Can you work these out from the model? Positions are in its coordinate system, mm. Face numbers are marked on the shaded views. A direction names the side the tool comes from. Round coordinates to 2 decimals unless told otherwise and drop trailing zeros. Write each loop counter-clockwise with the first axis right and the second up, starting at its lowest first coordinate (ties: lowest second). Pieces come first, ordered by that corner, then holes. Notation, with made-up numbers: M 88.25,-16 L 123.25,-16 A26 cw 123.25,8 Z; hole C 45.25,61 d4. An arc over 180 degrees is marked long. Answer in a Markdown table with one row per item. Add a question column.
(1) Suppose I cut it at B-B, the plane x = 3.5. Write out the boundary of the cut face in (y, z).
(2) If we mould it in two halves opening along Y, with no side actions, what happens to the marked faces 3, 4 and 5? For each: released by +Y, released by -Y, zero draft, split by the parting line, or undercut.
(3) I'm going to push flat-ended pins straight in: pin 1 (5.5 mm diameter, centred on x = 5, z = 28.5, fed in from +Y); pin 2 (10 mm diameter, centred on x = 29.5, z = 59.5, fed in from +Y); pin 3 (4 mm diameter, centred on y = 51, z = 30.5, fed in from +X); pin 4 (14 mm diameter, centred on x = 5.5, y = 52, fed in from -Z). Where does each tip first touch, or does it pass through?
(4) Suppose I cut it at C-C, the plane y = 37.5. Write out the boundary of the cut face in (x, z), then the cut area to 3 significant figures.
(5) For the marked faces 1 and 2, which set-ups out of +Z, -Z, +X, -X, +Y, -Y let a thin tool reach every point of the face, with its end or its side?
(6) If I drill on probe 1 along Z at (x, y) = (9.5, 28); probe 2 along X at (y, z) = (7, 19); probe 3 along Z at (x, y) = (7.5, 51), over which ranges is the centre line in solid material (lowest first)?
(7) Suppose I cut it at D-D, the plane x = 34. Write out the boundary of the cut face in (y, z).
(8) Suppose I cut it at A-A, the plane z = 31.5. Write out the boundary of the cut face in (x, y), then the cut area to 3 significant figures.
from build123d import *

# Parameters (mm, degrees)
SKETCH1_W           = 57.15
SKETCH1_H           = 57.15
BOSS_EXTRUDE1_DEPTH = 55.118
SKETCH2_R           = 19.05
BOSS_EXTRUDE2_DEPTH = 1.524
SKETCH3_R           = 3.175
BOSS_EXTRUDE3_DEPTH = 19.05
SKETCH18_W          = 20.32
SKETCH18_H          = 20.32
CUT_EXTRUDE13_DEPTH = 50.038
SKETCH20_W          = 20.32
SKETCH20_H          = 20.32
CUT_EXTRUDE14_DEPTH = 50.038
SKETCH21_W          = 20.32
SKETCH21_H          = 20.32
CUT_EXTRUDE15_DEPTH = 50.038
SKETCH22_W          = 20.32
SKETCH22_H          = 20.32
CUT_EXTRUDE16_DEPTH = 50.038
SKETCH11_R          = 2.54
CUT_EXTRUDE8_DEPTH  = 98.827597967
SKETCH12_R          = 2.54
CUT_EXTRUDE9_DEPTH  = 98.827597967
SKETCH14_R          = 2.54
CUT_EXTRUDE10_DEPTH = 98.827597967
SKETCH15_R          = 2.54
CUT_EXTRUDE11_DEPTH = 98.827597967
FILLET2_R           = 5.08
FILLET4_R           = 2.54
FILLET1_R           = 0.508
SKETCH10_W          = 7.148953117
SKETCH10_H          = 1.106198654
CUT_EXTRUDE7_DEPTH  = 14.986


with BuildPart() as part:
    # Sketch1 → Boss-Extrude1 (new body)
    with BuildSketch(Plane.XY):
        with Locations((28.575, 28.575)):
            Rectangle(SKETCH1_W, SKETCH1_H)
    extrude(amount=BOSS_EXTRUDE1_DEPTH)

    # Sketch2 → Boss-Extrude2 (add)
    with BuildSketch(Plane.XY.offset(55.118)):
        with Locations(Location((28.575, 28.575, 0), (0, 0, 180))):
            Circle(SKETCH2_R)
    extrude(amount=BOSS_EXTRUDE2_DEPTH)

    # Sketch3 → Boss-Extrude3 (add)
    with BuildSketch(Plane.XY.offset(56.642)):
        with Locations(Location((28.575, 28.575, 0), (0, 0, 180))):
            Circle(SKETCH3_R)
    extrude(amount=BOSS_EXTRUDE3_DEPTH)

    # Sketch18 → Cut-Extrude13 (cut)
    with BuildSketch(Plane(origin=(0, 0, 0), x_dir=(-1, 0, 0), z_dir=(0, 0, -1))):
        with Locations((0, 57.15)):
            Rectangle(SKETCH18_W, SKETCH18_H)
    extrude(amount=-CUT_EXTRUDE13_DEPTH, mode=Mode.SUBTRACT)

    # Sketch20 → Cut-Extrude14 (cut)
    with BuildSketch(Plane(origin=(0, 0, 0), x_dir=(-1, 0, 0), z_dir=(0, 0, -1))):
        Rectangle(SKETCH20_W, SKETCH20_H)
    extrude(amount=-CUT_EXTRUDE14_DEPTH, mode=Mode.SUBTRACT)

    # Sketch21 → Cut-Extrude15 (cut)
    with BuildSketch(Plane(origin=(0, 0, 0), x_dir=(-1, 0, 0), z_dir=(0, 0, -1))):
        with Locations((-57.15, 0)):
            Rectangle(SKETCH21_W, SKETCH21_H)
    extrude(amount=-CUT_EXTRUDE15_DEPTH, mode=Mode.SUBTRACT)

    # Sketch22 → Cut-Extrude16 (cut)
    with BuildSketch(Plane(origin=(0, 0, 0), x_dir=(-1, 0, 0), z_dir=(0, 0, -1))):
        with Locations((-57.15, 57.15)):
            Rectangle(SKETCH22_W, SKETCH22_H)
    extrude(amount=-CUT_EXTRUDE16_DEPTH, mode=Mode.SUBTRACT)

    # Sketch11 → Cut-Extrude8 (cut, through all)
    with BuildSketch(Plane.XY.offset(55.118)):
        with Locations((4.953, 52.233071325)):
            Circle(SKETCH11_R)
    extrude(amount=-CUT_EXTRUDE8_DEPTH, mode=Mode.SUBTRACT)

    # Sketch12 → Cut-Extrude9 (cut, through all)
    with BuildSketch(Plane.XY.offset(55.118)):
        with Locations((52.197, 52.233071325)):
            Circle(SKETCH12_R)
    extrude(amount=-CUT_EXTRUDE9_DEPTH, mode=Mode.SUBTRACT)

    # Sketch14 → Cut-Extrude10 (cut, through all)
    with BuildSketch(Plane.XY.offset(55.118)):
        with Locations((4.953, 4.989071325)):
            Circle(SKETCH14_R)
    extrude(amount=-CUT_EXTRUDE10_DEPTH, mode=Mode.SUBTRACT)

    # Sketch15 → Cut-Extrude11 (cut, through all)
    with BuildSketch(Plane.XY.offset(55.118)):
        with Locations((52.197, 4.989071325)):
            Circle(SKETCH15_R)
    extrude(amount=-CUT_EXTRUDE11_DEPTH, mode=Mode.SUBTRACT)

    # Fillet2
    fillet2_edges = [part.edges().sort_by_distance(p)[0] for p in [
        (0, 57.15, 52.578),
        (57.15, 57.15, 52.578),
        (57.15, 0, 52.578),
        (0, 0, 52.578),
    ]]
    fillet(fillet2_edges, radius=FILLET2_R)

    # Fillet4
    fillet4_edges = [part.edges().sort_by_distance(p)[0] for p in [
        (0, 28.575, 0),
        (10.16, 52.07, 0),
        (5.08, 46.99, 0),
        (0, 46.99, 25.019),
        (10.16, 57.15, 25.019),
        (10.16, 46.99, 25.019),
        (28.575, 0, 0),
        (5.08, 10.16, 0),
        (10.16, 5.08, 0),
        (10.16, 0, 25.019),
        (0, 10.16, 25.019),
        (10.16, 10.16, 25.019),
        (57.15, 28.575, 0),
        (46.99, 5.08, 0),
        (52.07, 10.16, 0),
        (57.15, 10.16, 25.019),
        (46.99, 0, 25.019),
        (46.99, 10.16, 25.019),
        (28.575, 57.15, 0),
        (52.07, 46.99, 0),
        (46.99, 52.07, 0),
        (46.99, 57.15, 25.019),
        (57.15, 46.99, 25.019),
        (46.99, 46.99, 25.019),
    ]]
    fillet(fillet4_edges, radius=FILLET4_R)

    # Fillet1
    fillet1_edges = [part.edges().sort_by_distance(p)[0] for p in [
        (31.75, 28.575, 75.692),
    ]]
    fillet(fillet1_edges, radius=FILLET1_R)

    # Sketch10 → Cut-Extrude7 (cut)
    with BuildSketch(Plane.XY.offset(75.692)):
        with Locations((29.031069878, 31.795099327)):
            Rectangle(SKETCH10_W, SKETCH10_H)
    extrude(amount=-CUT_EXTRUDE7_DEPTH, mode=Mode.SUBTRACT)


solid = part.part
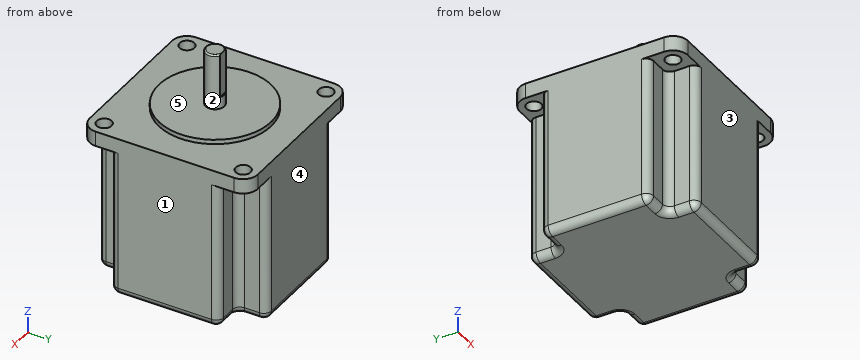
Calculated:
| question | item | result |
|---|---|---|
| 1 | outline | M 0.25,50.04 L 2.91,50.04 L 2.91,55.12 L 0.25,55.12 Z; M 7.07,50.04 L 10.16,50.04 L 10.16,2.54 A2.54 ccw 12.7,0 L 44.45,0 A2.54 ccw 46.99,2.54 L 46.99,50.04 L 50.15,50.04 L 50.15,55.12 L 7.07,55.12 Z; M 54.32,50.04 L 56.9,50.04 L 56.9,55.12 L 54.32,55.12 Z |
| 2 | face 3 | released by -Y |
| 2 | face 4 | released by +Y |
| 2 | face 5 | zero draft |
| 3 | pin 1 | y = 46.99 |
| 3 | pin 2 | y = 57.15 |
| 3 | pin 3 | x = 47.05 |
| 3 | pin 4 | z = 0.01 |
| 4 | outline | M 0,2.54 A2.54 ccw 2.54,0 L 54.61,0 A2.54 ccw 57.15,2.54 L 57.15,55.12 L 45.4,55.12 L 45.4,56.64 L 11.75,56.64 L 11.75,55.12 L 0,55.12 Z |
| 4 | area | 3,200 mm² |
| 5 | face 1 | +Z, -Z, +X, +Y, -Y |
| 5 | face 2 | +Z |
| 6 | probe 1 | 0 to 55.12 |
| 6 | probe 2 | 10.16 to 46.99 |
| 6 | probe 3 | 50.04 to 55.12 |
| 7 | outline | M 0,2.54 A2.54 ccw 2.54,0 L 54.61,0 A2.54 ccw 57.15,2.54 L 57.15,55.12 L 46.84,55.12 L 46.84,56.64 L 10.31,56.64 L 10.31,55.12 L 0,55.12 Z |
| 8 | outline | M 0,12.7 A2.54 ccw 2.54,10.16 L 7.62,10.16 A2.54 cw 10.16,7.62 L 10.16,2.54 A2.54 ccw 12.7,0 L 44.45,0 A2.54 ccw 46.99,2.54 L 46.99,7.62 A2.54 cw 49.53,10.16 L 54.61,10.16 A2.54 ccw 57.15,12.7 L 57.15,44.45 A2.54 ccw 54.61,46.99 L 49.53,46.99 A2.54 cw 46.99,49.53 L 46.99,54.61 A2.54 ccw 44.45,57.15 L 12.7,57.15 A2.54 ccw 10.16,54.61 L 10.16,49.53 A2.54 cw 7.62,46.99 L 2.54,46.99 A2.54 ccw 0,44.45 Z |
| 8 | area | 2,850 mm² |
